Work out the finished part from the listing and answer in its coordinate system (mm). A direction names the side the tool comes from. Round coordinates to 2 decimals unless told otherwise and drop trailing zeros. Order: outer loops, then holes, each group sorted by start corner. A loop starts at its lowest first (then second) coordinate and runs counter-clockwise, first axis right, second up. Notation, with made-up numbers: (41, 64.5) - (82, 64.5) arc R20 ccw to (82, 70.5) - close; hole circle Ø6 at (62, 4). An arc over 180 degrees is marked (long way). Use CSV: the item, a comma, the result in double quotes.
from build123d import *

# Parameters (mm, degrees)
F1_DEPTH = 1
F2_R     = 0.2


with BuildPart() as f1:
    # F0 (on Front) → F1 (new body)
    with BuildSketch(Plane.XZ):
        with BuildLine():
            Line((2.8, 0), (2, 0))
            ThreePointArc((2, 0), (1.870829, -0.707107), (1.5, -1.322876))
            Line((1.5, -1.322876), (2.2, -3.925557))
            ThreePointArc((2.2, -3.925557), (3.882654, -2.274863), (4.5, 0))
            ThreePointArc((4.5, 0), (-2.274863, 3.882654), (-2.2, -3.925557))
            Line((-2.2, -3.925557), (-1.5, -1.322876))
            ThreePointArc((-1.5, -1.322876), (-1.870829, -0.707107), (-2, 0))
            Line((-2, 0), (-2.8, 0))
            ThreePointArc((-2.8, 0), (-2.366384, 1.495757), (-1.2, 2.527677))
            Line((-1.2, 2.527677), (-0.9, 1.786057))
            ThreePointArc((-0.9, 1.786057), (0, 2), (0.9, 1.786057))
            Line((0.9, 1.786057), (1.2, 2.527677))
            ThreePointArc((1.2, 2.527677), (2.366384, 1.495757), (2.8, 0))
        make_face()
    extrude(amount=F1_DEPTH)

    # F2
    f2_edges = [f1.edges().sort_by_distance(p)[0] for p in [
        (-1.2, -0.5, 2.527677),
        (1.2, -0.5, 2.527677),
        (2.8, -0.5, 0),
        (-2.8, -0.5, 0),
    ]]
    fillet(f2_edges, radius=F2_R)


solid = f1.part
(1) Find section B-B (x = -1.75). Determine the outline of the cut face in (y, z), and give its area (3 significant figures).
Findings below:
outline,"(-1, -2.25) - (0, -2.25) - (0, -0.97) - (-1, -0.97) - close; (-1, 2.18) - (0, 2.18) - (0, 4.15) - (-1, 4.15) - close"
area,"3.25 mm²"
(2) For faces 1 (the cylindrical face through (1.874, -0.493, -0.698)), 2 (the flat face through (-0.1, 0, 2.2)), 3 (the flat face through (-1.855, -0.493, -2.642)), determine the directions among +Z, -Z, +X, -X, +Y, -Y from which every point of the face is accessible in a straight line to the end or side of a thin tool.
Findings below:
face 1,"+Y, -Y"
face 2,"+Z, -Z, +X, -X, +Y"
face 3,"-Z, +Y, -Y"
(3) Find section A-A (z = -0.25). Determine the outline of the cut face in (x, y), and give its area (3 significant figures).
Findings below:
outline,"(-4.49, -1) - (-1.98, -1) - (-1.98, 0) - (-4.49, 0) - close; (1.98, -1) - (4.49, -1) - (4.49, 0) - (1.98, 0) - close"
area,"5.02 mm²"
(4) Find the intervals of material crossed by L1, parallel to X at y = -0.2, z = 1.75; L2, parallel to X at y = -0.55, z = 0.25; L3, parallel to Z at x = 2.5, y = -0.1, in increasing order. Write a range as from..to.
Findings below:
L1,"x = -4.15..-2.18, 2.18..4.15"
L2,"x = -4.49..-2.79, 2.79..4.49"
L3,"z = -3.74..0, 1.26..3.74"
(5) This flat-tipped pin is pushed along its axis until it touches: pin 1 (0.5 mm diameter, centred on x = -2.5, y = -0.5, fed in from +Z). Where does it stop, or does it pass through?
Findings below:
pin 1,"stops at z = 3.9"
(6) The mould has two halves that part along Z. Classify faces 4 (the cylindrical face through (-2.38, -0.493, 1.474)), 5 (the flat face through (-0.1, -1, 2.2)), 6 (the cylindrical face through (0, -0.5, 2)), 7 (the cylindrical face through (2.36, -0.493, 1.506)): released by +Z, released by -Z, zero draft, split by the parting line, or undercut.
Findings below:
face 4,"undercut"
face 5,"zero draft"
face 6,"released by -Z"
face 7,"undercut"
(7) Find section C-C (y = -0.6). Determine the outline of the cut face in (x, z).
Findings below:
outline,"(-2.79, 0.22) arc R2.8 cw to (-1.4, 2.42) arc R0.2 cw to (-1.12, 2.32) - (-0.9, 1.79) arc R2 cw to (0.9, 1.79) - (1.12, 2.32) arc R0.2 cw to (1.4, 2.42) arc R2.8 cw to (2.79, 0.22) arc R0.2 cw to (2.59, 0) - (2, 0) arc R2 cw to (1.5, -1.32) - (2.2, -3.93) arc R4.5 ccw to (4.5, 0) arc R4.5 ccw (long way) to (-2.2, -3.93) - (-1.5, -1.32) arc R2 cw to (-2, 0) - (-2.59, 0) arc R0.2 cw to start"
(8) Find section D-D (x = 0). Determine the outline of the cut face in (y, z), and give its area (3 significant figures).
Findings below:
outline,"(-1, 2) - (0, 2) - (0, 4.5) - (-1, 4.5) - close"
area,"2.50 mm²"
